Read the model definition and answer for the solid it produces. Units are mm, in the model's axes. A direction names the side the tool comes from. Round coordinates to 2 decimals unless told otherwise and drop trailing zeros. Write each loop counter-clockwise with the first axis right and the second up, starting at its lowest first coordinate (ties: lowest second). Pieces come first, ordered by that corner, then holes. Notation, with made-up numbers: (50, 86) - (70, 86) arc R24 ccw to (70, 113) - close; hole circle Ø2 at (1.25, 40.25). An arc over 180 degrees is marked (long way). Use one line per item in the form item = value. Start each with the question number.
1) The part is cut by section B-B, the plane y = 3. Give the vertices of the cut face in (x, z).
2) For faces 1 (the face through (3.73, -7.58, -23.59)), 2 (the face through (14, -9, 6.455)), 3 (the face through (3, -12, -29.2)), determine the directions among +Z, -Z, +X, -X, +Y, -Y from which every point of the face is accessible in a straight line to the end or side of a thin tool.
3) The part is cut by section D-D, the plane y = -8.5. Give the vertices of the cut face in (x, z).
4) For a pull along Y with two mould halves and no side action, classify faces 4 (the face through (5, -14.1, 20)), 5 (the face through (-13.6, 1.4, 2)), 6 (the face through (12.885, 0.045, 0.986)) as released by +Y, released by -Y, zero draft, split by the parting line, or undercut.
5) Each of these flat-tipped pins is pushed along its axis until it touches: pin 1 (4.5 mm diameter, centred on x = 3.5, z = -19.5, fed in from +Y); pin 2 (8 mm diameter, centred on y = -12, z = -1.5, fed in from +X); pin 3 (15 mm diameter, centred on x = 4.75, z = -19, fed in from -Y); pin 4 (2 mm diameter, centred on x = -10.5, y = -1.5, fed in from -Z). Where does it stop, or does it pass through?
6) Consider line 1 along Y through (x, z) = (13.9, 0.9); line 2 along X through (y, z) = (1.75, 1.5); line 3 along Y through (x, z) = (4.5, -9). Determine where each line is inside the solid, lowest interval first. Write a range as from..to.
7) The part is cut by section C-C, the plane x = -13.9. Give the vertices of the cut face in (y, z).
8) The part is cut by section A-A, the plane z = -19. Give the vertices of the cut face in (x, y).
from build123d import *

# Parameters (mm, degrees)
SKETCH1_R           = 1.016
BOSS_EXTRUDE1_DEPTH = 2
SKETCH2_R           = 4.7
BOSS_EXTRUDE2_DEPTH = 3
BOSS_EXTRUDE5_DEPTH = 8
BOSS_EXTRUDE6_START = -27.3
BOSS_EXTRUDE6_DEPTH = 32.1
SKETCH4_W           = 22.5
SKETCH4_H           = 14.127681706
CUT_EXTRUDE1_DEPTH  = 7
FILLET1_R           = 0.5
SKETCH5_R           = 2.5
BOSS_EXTRUDE7_DEPTH = 1
SKETCH6_W           = 5.313656685
SKETCH6_H           = 4.599259183
SKETCH6_W_2         = 16.163165117
SKETCH6_H_2         = 5.344557169
CUT_EXTRUDE2_DEPTH  = 5


with BuildPart() as part:
    # Sketch1 → Boss-Extrude1 (new body)
    # profile 1 of 4: a face of its own
    with BuildSketch(Plane.XY):
        with BuildLine():
            Line((-16.05, 5.25), (-16.05, -5.25))
            ThreePointArc((-16.05, -5.25), (-15.801040764, -5.851040764), (-15.2, -6.1))
            Line((-15.2, -6.1), (-11.25, -6.1))
            Line((-11.25, -6.1), (-11.25, 6.1))
            Line((-11.25, 6.1), (-15.2, 6.1))
            ThreePointArc((-15.2, 6.1), (-15.801040764, 5.851040764), (-16.05, 5.25))
        make_face()
        with Locations((-13.9, 0)):
            Circle(SKETCH1_R, mode=Mode.SUBTRACT)
    # profile 2 of 4: a face of its own
    with BuildSketch(Plane.XY):
        with BuildLine():
            Line((16.05, 5.25), (16.05, -5.25))
            ThreePointArc((16.05, -5.25), (15.801040764, -5.851040764), (15.2, -6.1))
            Line((15.2, -6.1), (11.25, -6.1))
            Line((11.25, -6.1), (11.25, 6.094097151))
            Line((11.25, 6.094097151), (15.2, 6.1))
            ThreePointArc((15.2, 6.1), (15.801040764, 5.851040764), (16.05, 5.25))
        make_face()
        with Locations((13.9, 0)):
            Circle(SKETCH1_R, mode=Mode.SUBTRACT)
    # profile 3 of 4: a face of its own
    with BuildSketch(Plane.XY):
        with BuildLine():
            ThreePointArc((15.2, -6.1), (15.801040764, -5.851040764), (16.05, -5.25))
            Line((16.05, -5.25), (16.05, -6.1))
            Line((16.05, -6.1), (15.2, -6.1))
        make_face()
    # profile 4 of 4: a face of its own
    with BuildSketch(Plane.XY):
        with BuildLine():
            ThreePointArc((-16.05, -5.25), (-15.801040764, -5.851040764), (-15.2, -6.1))
            Line((-15.2, -6.1), (-16.05, -6.1))
            Line((-16.05, -6.1), (-16.05, -5.25))
        make_face()
    extrude(amount=BOSS_EXTRUDE1_DEPTH)

    # Sketch2 → Boss-Extrude2 (add)
    with BuildSketch(Plane.XZ.offset(6.1)):
        Polygon((16.05, 2), (11.25, 2), (11.25, 18.429366849), (-1.65, 23.613902023), (-1.65, 2), (-16.05, 2), (-16.05, 0), (-1.65, 0), (-1.65, -29.999830432), (11.25, -29.999830432), (11.25, 0), (16.05, 0), align=None)
        with Locations((4.75, -19)):
            Circle(SKETCH2_R, mode=Mode.SUBTRACT)
    extrude(amount=BOSS_EXTRUDE2_DEPTH)

    # Sketch2<3> → Boss-Extrude5 (add)
    with BuildSketch(Plane.XZ.offset(6.1)):
        with BuildLine():
            ThreePointArc((8.578413339, 18.144332102), (9.979514579, 17.458386729), (11.25, 16.553139508))
            Line((11.25, 16.553139508), (11.25, 18.429366849))
            Line((11.25, 18.429366849), (-1.65, 23.613902023))
            Line((-1.65, 23.613902023), (-1.65, 22.612965014))
            Line((-1.65, 22.612965014), (-1.57491206, 22.257159966))
            Line((-1.57491206, 22.257159966), (8.578413339, 18.144332102))
        make_face()
        with BuildLine():
            ThreePointArc((0.350023778, -29.2), (-0.651218811, -29.175170712), (-1.65, -29.100743889))
            Line((-1.65, -29.100743889), (-1.65, -29.999830432))
            Line((-1.65, -29.999830432), (11.25, -29.999830432))
            Line((11.25, -29.999830432), (11.25, -26.86066155))
            ThreePointArc((11.25, -26.86066155), (8.204073841, -28.597362862), (4.75, -29.2))
            Line((4.75, -29.2), (0.350023778, -29.2))
        make_face()
    extrude(amount=BOSS_EXTRUDE5_DEPTH)

    # Sketch3 → Boss-Extrude6 (add)
    with BuildSketch(Plane(origin=(11.25, 0, 0), x_dir=(0, 0, -1), z_dir=(1, 0, 0)).offset(BOSS_EXTRUDE6_START)):
        Polygon((-7.665828596, -9.1), (-2, -3.457464127), (-2, -9.1), align=None)
    extrude(amount=BOSS_EXTRUDE6_DEPTH)

    # Sketch4 → Cut-Extrude1 (cut)
    with BuildSketch(Plane(origin=(0, -6.1, 0), x_dir=(1, 0, 0), z_dir=(0, 1, 0))):
        with Locations((0, -7.063840853)):
            Rectangle(SKETCH4_W, SKETCH4_H)
    extrude(amount=CUT_EXTRUDE1_DEPTH, mode=Mode.SUBTRACT)

    # Fillet1
    fillet1_edges = [part.edges().sort_by_distance(p)[0] for p in [
        (13.65, -9.1, 7.665828596),
        (-8.85, -9.1, 7.665828596),
    ]]
    fillet(fillet1_edges, radius=FILLET1_R)

    # Sketch5 → Boss-Extrude7 (add)
    with BuildSketch(Plane.XZ.offset(9.1)):
        with BuildLine():
            Line((-1.65, 22.612965014), (-1.65, 6.455196792))
            Line((-1.65, 6.455196792), (-16.05, 6.455196792))
            Line((-16.05, 6.455196792), (-16.05, 0))
            Line((-16.05, 0), (-1.65, 0))
            Line((-1.65, 0), (-1.65, -29.100743889))
            ThreePointArc((-1.65, -29.100743889), (-0.651218811, -29.175170712), (0.350023778, -29.2))
            Line((0.350023778, -29.2), (4.75, -29.2))
            ThreePointArc((4.75, -29.2), (8.204073841, -28.597362862), (11.25, -26.86066155))
            Line((11.25, -26.86066155), (11.25, 0))
            Line((11.25, 0), (16.05, 0))
            Line((16.05, 0), (16.05, 6.455196792))
            Line((16.05, 6.455196792), (11.25, 6.455196792))
            Line((11.25, 6.455196792), (11.25, 16.553139508))
            ThreePointArc((11.25, 16.553139508), (9.979514579, 17.458386729), (8.578413339, 18.144332102))
            Line((8.578413339, 18.144332102), (-1.57491206, 22.257159966))
            Line((-1.57491206, 22.257159966), (-1.65, 22.612965014))
        make_face()
        with Locations((4.75, -19)):
            Circle(SKETCH5_R, mode=Mode.SUBTRACT)
    extrude(amount=BOSS_EXTRUDE7_DEPTH)

    # Sketch6 → Cut-Extrude2 (cut)
    with BuildSketch(Plane.XY.offset(6.455196792)):
        with Locations((13.906828343, -7.800370409)):
            Rectangle(SKETCH6_W, SKETCH6_H)
        with Locations((-9.731582558, -7.427721416)):
            Rectangle(SKETCH6_W_2, SKETCH6_H_2)
    extrude(amount=CUT_EXTRUDE2_DEPTH, mode=Mode.SUBTRACT)


solid = part.part
Geometry results:
q1.outline = (-16.05, 0) - (-11.25, 0) - (-11.25, 2) - (-16.05, 2) - close; (11.25, 0) - (16.05, 0) - (16.05, 2) - (11.25, 2) - close
q2.face_1 = +Y
q2.face_2 = +Z, +X, +Y, -Y
q2.face_3 = -Y
q3.outline = (-16.05, 0) - (-1.65, 0) - (-1.65, -30) - (11.25, -30) - (11.25, 0) - (16.05, 0) - (16.05, 6.46) - (11.25, 6.46) - (11.25, 18.43) - (-1.65, 23.61) - (-1.65, 6.46) - (-16.05, 6.46) - close; hole circle Ø9.4 at (4.75, -19)
q4.face_4 = released by -Y
q4.face_5 = zero draft
q4.face_6 = undercut
q5.pin_1 = -9.1
q5.pin_2 = 16.05
q5.pin_3 = -10.1
q5.pin_4 = 0
q6.line_1 = -10.1..-1.02, 1.02..6.1
q6.line_2 = -16.05..-11.25, 11.25..16.05
q6.line_3 = -10.1..-6.1
q7.outline = (-10.1, 0) - (-1.02, 0) - (-1.02, 2) - (-3.46, 2) - (-7.89, 6.46) - (-10.1, 6.46) - close; (1.02, 0) - (6.1, 0) - (6.1, 2) - (1.02, 2) - close
q8.outline = (-1.65, -10.1) - (2.25, -10.1) - (2.25, -9.1) - (0.05, -9.1) - (0.05, -6.1) - (-1.65, -6.1) - close; (7.25, -10.1) - (11.25, -10.1) - (11.25, -6.1) - (9.45, -6.1) - (9.45, -9.1) - (7.25, -9.1) - close
